Verification items for this drawing (mm, ordinates from the low corner). Coordinates: 2 decimals unless noted, no trailing zeros. Order: outer loops, then holes, each group sorted by start corner. A loop starts at its lowest first (then second) coordinate and runs counter-clockwise, first axis right, second up.
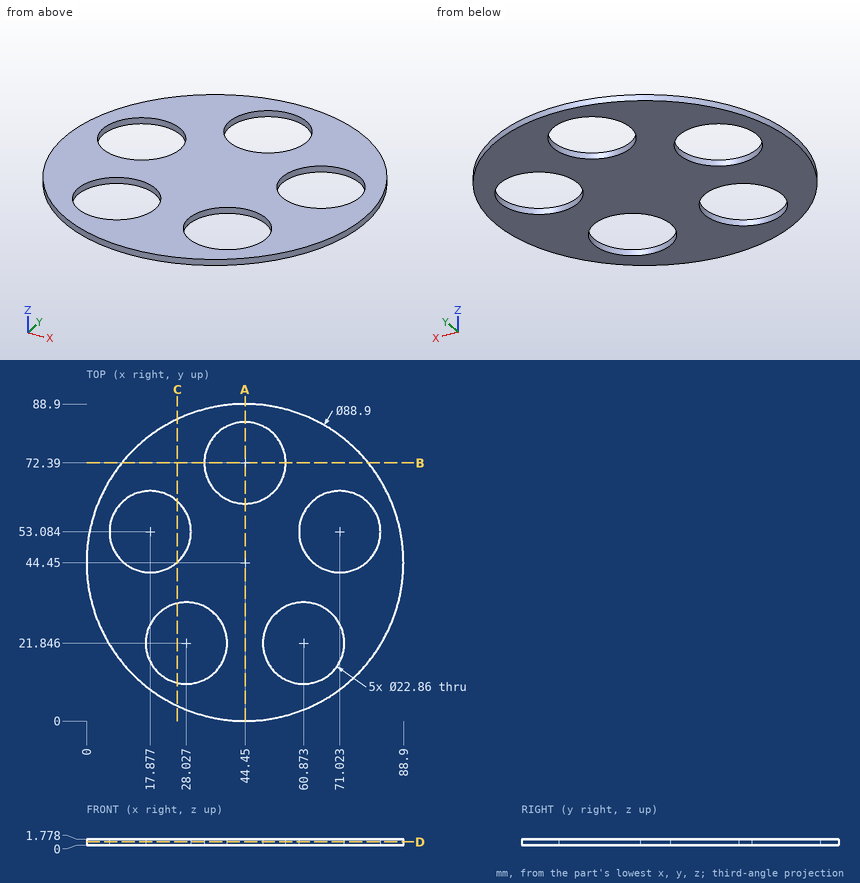
Item 1: Sectioned sample at C-C (x = 25.5). Record the cut outline in (y, z).
Item 2: Sectioned sample at D-D (z = 1). Record the cut outline in (x, y).
Item 3: Sectioned sample at A-A (x = 44.45). Record the cut outline in (y, z).
Item 4: Thickness scan on line 1 along Y through (x, z) = (61, 1.15) (1 decimal); line 2 along Y through (x, z) = (44.45, 1.1); line 3 along X through (y, z) = (30.5, 1.35) (1 decimal). Record the ranges inside material, lowest first.
Item 5: Sectioned sample at B-B (y = 72.39). Record the cut outline in (x, z).
Item 6: Depth check by flat-ended pin: P1, Ø13.5, axis at x = 28.03, y = 21.85, coming from the -Z side; P2, Ø1, axis at y = 41, z = 0.5, coming from the +X side. Enter the tip coordinate at first touch or a pass-through.
Geometry check:
1. outline: (4.24, 0) - (10.7, 0) - (10.7, 1.78) - (4.24, 1.78) - close; (32.99, 0) - (44.57, 0) - (44.57, 1.78) - (32.99, 1.78) - close; (61.6, 0) - (84.66, 0) - (84.66, 1.78) - (61.6, 1.78) - close
2. outline: circle Ø88.9 at (44.45, 44.45); hole circle Ø22.86 at (17.88, 53.08); hole circle Ø22.86 at (28.03, 21.85); hole circle Ø22.86 at (44.45, 72.39); hole circle Ø22.86 at (60.87, 21.85); hole circle Ø22.86 at (71.02, 53.08)
3. outline: (0, 0) - (60.96, 0) - (60.96, 1.78) - (0, 1.78) - close; (83.82, 0) - (88.9, 0) - (88.9, 1.78) - (83.82, 1.78) - close
4. line 1: y = 3.2 to 10.4, 33.3 to 47.6, 58.6 to 85.7
4. line 2: y = 0 to 60.96, 83.82 to 88.9
4. line 3: x = 2.2 to 20.6, 35.5 to 53.4, 68.3 to 86.7
5. outline: (9.88, 0) - (33.02, 0) - (33.02, 1.78) - (9.88, 1.78) - close; (55.88, 0) - (79.02, 0) - (79.02, 1.78) - (55.88, 1.78) - close
6. P1: passes through
6. P2: stops at x = 88.8
